Model file for the job. Use its own axes, mm. Face numbers are marked on the shaded views. A direction names the side the tool comes from. Coordinates: 2 decimals unless noted, no trailing zeros. Write each loop counter-clockwise with the first axis right and the second up, starting at its lowest first coordinate (ties: lowest second). Pieces come first, ordered by that corner, then holes. Notation, with made-up numbers: M -11.5,60 L 28.5,60 A19 cw 28.5,76 Z; hole C -23.75,-25 d11. An arc over 180 degrees is marked long. Use CSV: the item, a comma, the result in double quotes. Start each with the question number.
from build123d import *

# Parameters (mm, degrees)
BOSS_EXTRUDE1_DEPTH  = 50
SKETCH2_W            = 150
SKETCH2_H            = 10
BOSS_EXTRUDE2_DEPTH  = 400
SKETCH3_W            = 400
SKETCH3_H            = 10
BOSS_EXTRUDE3_DEPTH  = 446
MIRROR2_COPY_1_DEPTH = 50
SKETCH4_W            = 111.615994823
SKETCH4_H            = 184.082968076
BOSS_EXTRUDE4_DEPTH  = 100
SKETCH5_R            = 14.792808223
SKETCH5_R_2          = 5.397690937
BOSS_EXTRUDE5_DEPTH  = 5


with BuildPart() as part:
    # Sketch1 → Boss-Extrude1 (new body)
    with BuildSketch(Plane.XY):
        with BuildLine():
            ThreePointArc((-54, 0), (0, 54), (54, 0))
            Line((54, 0), (75, 0))
            ThreePointArc((75, 0), (0, 75), (-75, 0))
            Line((-75, 0), (-54, 0))
        make_face()
    boss_extrude1 = extrude(amount=BOSS_EXTRUDE1_DEPTH)

    # Sketch2 → Boss-Extrude2 (add)
    with BuildSketch(Plane(origin=(0, 0, 0), x_dir=(-1, 0, 0), z_dir=(0, 0, -1))):
        with Locations((0, 5)):
            Rectangle(SKETCH2_W, SKETCH2_H)
    extrude(amount=BOSS_EXTRUDE2_DEPTH)

    # Mirror1: Boss-Extrude1 across plane
    add(boss_extrude1.mirror(Plane(origin=(0, 0, -200), x_dir=(1, 0, 0), z_dir=(0, 0, -1))))

    # Sketch3 → Boss-Extrude3 (add)
    with BuildSketch(Plane(origin=(75, 0, 0), x_dir=(0, 0, -1), z_dir=(1, 0, 0))):
        with Locations((200, 5)):
            Rectangle(SKETCH3_W, SKETCH3_H)
    extrude(amount=BOSS_EXTRUDE3_DEPTH)

    # Mirror2: Boss-Extrude1 across plane
    add(boss_extrude1.mirror(Plane.ZY.offset(-223)))

    # Mirror2 copy 1 sketch → Mirror2 copy 1 (add)
    with BuildSketch(Plane(origin=(446, 0, -400), x_dir=(-1, 0, 0), z_dir=(0, 0, -1))):
        with BuildLine():
            ThreePointArc((-54, 0), (0, 54), (54, 0))
            Line((54, 0), (75, 0))
            ThreePointArc((75, 0), (0, 75), (-75, 0))
            Line((-75, 0), (-54, 0))
        make_face()
    extrude(amount=MIRROR2_COPY_1_DEPTH)

    # Sketch4 → Boss-Extrude4 (add)
    with BuildSketch(Plane(origin=(0, 10, 0), x_dir=(1, 0, 0), z_dir=(0, 1, 0))):
        with Locations((465.192002589, 243.791802991)):
            Rectangle(SKETCH4_W, SKETCH4_H)
    extrude(amount=BOSS_EXTRUDE4_DEPTH)

    # Sketch5 → Boss-Extrude5 (add)
    # profile 1 of 3: a face of its own
    with BuildSketch(Plane(origin=(521, 0, 0), x_dir=(0, 0, -1), z_dir=(1, 0, 0))):
        with Locations(Location((212.154840545, 79.041859429, 0), (0, 0, 180))):
            Circle(SKETCH5_R)
        with Locations((212.154840545, 79.041859429)):
            Circle(SKETCH5_R_2, mode=Mode.SUBTRACT)
    # profile 2 of 3: a face of its own
    with BuildSketch(Plane(origin=(521, 0, 0), x_dir=(0, 0, -1), z_dir=(1, 0, 0))):
        with Locations(Location((278.712975673, 79.041859429, 0), (0, 0, 180))):
            Circle(SKETCH5_R)
        with Locations((278.712975673, 79.041859429)):
            Circle(SKETCH5_R_2, mode=Mode.SUBTRACT)
    # profile 3 of 3: a face of its own
    with BuildSketch(Plane(origin=(521, 0, 0), x_dir=(0, 0, -1), z_dir=(1, 0, 0))):
        with BuildLine():
            Line((280.00330423, 50.703730269), (286.391115278, 47.708316048))
            ThreePointArc((286.391115278, 47.708316048), (248.501595961, 21.641542626), (207.227203105, 41.927420598))
            Line((207.227203105, 41.927420598), (213.112092722, 45.819041152))
            ThreePointArc((213.112092722, 45.819041152), (247.987758497, 28.678062178), (280.00330423, 50.703730269))
        make_face()
    extrude(amount=BOSS_EXTRUDE5_DEPTH)


solid = part.part
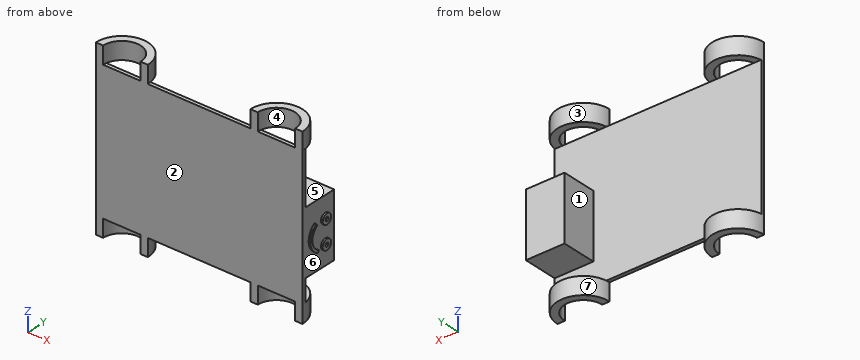
1) Tool access for the marked faces 3, 4, 5, 6 and 7: list every direction of +Z, -Z, +X, -X, +Y, -Y with a clear straight run to the whole face (end or side of a thin tool).
2) Band-saw the part on C-C on z = -349. List the corners of the cut face in (x, y), then the cut area to 3 significant figures.
3) Drop flat-ended pins along their axis: P1, Ø3, axis at x = 14.5, y = 4, coming from the +Z side; P2, Ø5.5, axis at y = 80.5, z = -278.5, coming from the +X side; P3, Ø11, axis at x = 458, y = 7, coming from the -Z side. Give the stop position or say it passes through.
4) Wall check: L1, parallel to Z at x = 494.5, y = 38; L2, parallel to Z at x = -17.5, y = 61; L3, parallel to X at y = 46, z = -306. Give the ranges that are in metal, low to high. Write a range as [from, to].
5) Band-saw the part on D-D on x = 291. List the corners of the cut face in (y, z).
6) Band-saw the part on A-A on x = 0. List the corners of the cut face in (y, z), then the cut area to 3 significant figures.
7) Two-plate mould, pull along Z, no slides. Class the marked faces 1 and 2: pulls with the +Z half, pulls with the -Z half, needs draft (parallel to the pull), parting line crosses it, or undercut.
8) Band-saw the part on B-B on x = 446. List the corners of the cut face in (y, z), then the cut area to 3 significant figures.
Findings below:
1,face 3,"+Z, +Y"
1,face 4,"+Z, -Y"
1,face 5,"+X, -X, +Y"
1,face 6,"+X"
1,face 7,"-Z, +Y"
2,outline,"M -75,0 L 521,0 L 521,10 L -75,10 Z"
2,area,"5,960 mm2"
3,P1,"stops at z = 0"
3,P2,"stops at x = 521"
3,P3,"stops at z = -400"
4,L1,"z = [-450, -400], [-335.83, -151.75], [0, 50]"
4,L2,"z = [-450, -400], [0, 50]"
4,L3,"x = [409.38, 521]"
5,outline,"M 0,-400 L 10,-400 L 10,0 L 0,0 Z"
6,outline,"M 0,-400 L 10,-400 L 10,0 L 0,0 Z; M 54,-450 L 75,-450 L 75,-400 L 54,-400 Z; M 54,0 L 75,0 L 75,50 L 54,50 Z"
6,area,"6,100 mm2"
7,face 1,"undercut"
7,face 2,"needs draft"
8,outline,"M 0,-400 L 10,-400 L 10,-335.83 L 110,-335.83 L 110,-151.75 L 10,-151.75 L 10,0 L 0,0 Z; M 54,-450 L 75,-450 L 75,-400 L 54,-400 Z; M 54,0 L 75,0 L 75,50 L 54,50 Z"
8,area,"24,500 mm2"
